Build history of the part. All positions in model axes, mm. A direction names the side the tool comes from. Give positions to 0.01 mm unless a question says otherwise; leave off trailing zeros. Order: outer loops, then holes, each group sorted by start corner. A loop starts at its lowest first (then second) coordinate and runs counter-clockwise, first axis right, second up. Notation, with made-up numbers: (24, 79) - (72, 79) arc R31 cw to (72, 108) - close; hole circle Ø5 at (48.25, 6.25). An arc over 180 degrees is marked (long way). Use a Markdown table: item, result. Add a question column.
(1) Slice it at D-D (x = 27). Write the cut outline in (y, z), then the cut area to 3 significant figures.
(2) Slice it at B-B (x = -12.5). Write the cut outline in (y, z), then the cut area to 3 significant figures.
(3) Flat gauge pins, fed straight in: pin 1 (1.5 mm diameter, centred on y = 13.5, z = 1.5, fed in from -X); pin 2 (1.5 mm diameter, centred on x = -12, y = -13, fed in from +Z); pin 3 (3 mm diameter, centred on x = 20.5, z = 3, fed in from -Y). Where does each tip first touch, or does it go through?
(4) Which spindle directions (+Z, -Z, +X, -X, +Y, -Y) get a long thin tool onto all of the face, cutting with end or side? Do faces 1 (the face through (11, -12.43, 4.01)), 2 (the face through (11.95, -11.99, 1.52)). Say none if no direction does.
(5) Mould opens along X. For faces 3 (the face through (31, 9.76, 2.46)), 4 (the face through (0, 0, 0)), 5 (the face through (-14, 12.57, 4.01)) say: +X half, -X half, draft (parallel to the pull), parting line (faces both ways), or undercut.
(6) Wall check: line 1 (Y direction, x = 12.5, z = 4.35); line 2 (Y direction, x = 12.5, z = 1.35); line 3 (X direction, y = 14.5, z = 1.1). Give the ranges that are in metal, low to high.
(7) Slice it at C-C (z = 4.1). Write the cut outline in (x, y), then the cut area to 3 significant figures.
(8) Slice it at A-A (y = -12.5). Write the cut outline in (x, z), then the cut area to 4 significant figures.
from build123d import *

# Parameters (mm, degrees)
F0_R     = 32.5
F1_DEPTH = 5
F4_R     = 0.75
F4_R_2   = 1
F5_DEPTH = 5
F3_R     = 1.5
F6_DEPTH = 2


with BuildPart() as f1:
    # F0 (on Top) → F1 (new body)
    with BuildSketch(Plane.XY):
        Circle(F0_R)
    extrude(amount=F1_DEPTH)

    # F4 (on face) → F5 (cut)
    with BuildSketch(Plane.XY.offset(5)):
        with Locations((12.5, -12.5)):
            Circle(F4_R)
        with Locations((-12.5, 12.5)):
            Circle(F4_R_2)
        with Locations((-12.5, -12.5)):
            Circle(F4_R_2)
        with Locations((12.5, 12.5)):
            Circle(F4_R_2)
    extrude(amount=-F5_DEPTH, mode=Mode.SUBTRACT)

    # F3 (on face) → F6 (cut)
    with BuildSketch(Plane.XY.offset(5)):
        with Locations((12.5, 12.5)):
            Circle(F3_R)
        with Locations((12.5, -12.5)):
            Circle(F3_R)
        with Locations((-12.5, -12.5)):
            Circle(F3_R)
        with Locations((-12.5, 12.5)):
            Circle(F3_R)
    extrude(amount=-F6_DEPTH, mode=Mode.SUBTRACT)


solid = f1.part
Solution:
| question | item | result |
|---|---|---|
| 1 | outline | (-18.09, 0) - (18.09, 0) - (18.09, 5) - (-18.09, 5) - close |
| 1 | area | 181 mm2 |
| 2 | outline | (-30, 0) - (-13.5, 0) - (-13.5, 3) - (-14, 3) - (-14, 5) - (-30, 5) - close; (-11.5, 0) - (11.5, 0) - (11.5, 3) - (11, 3) - (11, 5) - (-11, 5) - (-11, 3) - (-11.5, 3) - close; (13.5, 0) - (30, 0) - (30, 5) - (14, 5) - (14, 3) - (13.5, 3) - close |
| 2 | area | 276 mm2 |
| 3 | pin 1 | x = -29.89 |
| 3 | pin 2 | z = 3 |
| 3 | pin 3 | y = -26.37 |
| 4 | face 1 | +Z |
| 4 | face 2 | +Z, -Z |
| 5 | face 3 | parting line |
| 5 | face 4 | draft |
| 5 | face 5 | undercut |
| 6 | line 1 | -30 to -14, -11 to 11, 14 to 30 |
| 6 | line 2 | -30 to -13.25, -11.75 to 11.5, 13.5 to 30 |
| 6 | line 3 | -29.09 to 29.09 |
| 7 | outline | circle Ø65 at (0, 0); hole circle Ø3 at (-12.5, -12.5); hole circle Ø3 at (-12.5, 12.5); hole circle Ø3 at (12.5, -12.5); hole circle Ø3 at (12.5, 12.5) |
| 7 | area | 3,290 mm2 |
| 8 | outline | (-30, 0) - (-13.5, 0) - (-13.5, 3) - (-14, 3) - (-14, 5) - (-30, 5) - close; (-11.5, 0) - (11.75, 0) - (11.75, 3) - (11, 3) - (11, 5) - (-11, 5) - (-11, 3) - (-11.5, 3) - close; (13.25, 0) - (30, 0) - (30, 5) - (14, 5) - (14, 3) - (13.25, 3) - close |
| 8 | area | 277.5 mm2 |
